Geometry check sheet. Reference: drawing and pictorial views, mm from the part's lowest x, y, z. A direction names the side the tool comes from. Coordinates: 2 decimals unless noted, no trailing zeros. Loops run counter-clockwise (first coordinate to the right, second up) from the corner with the lowest first, then second, coordinate; pieces in that order, holes last.
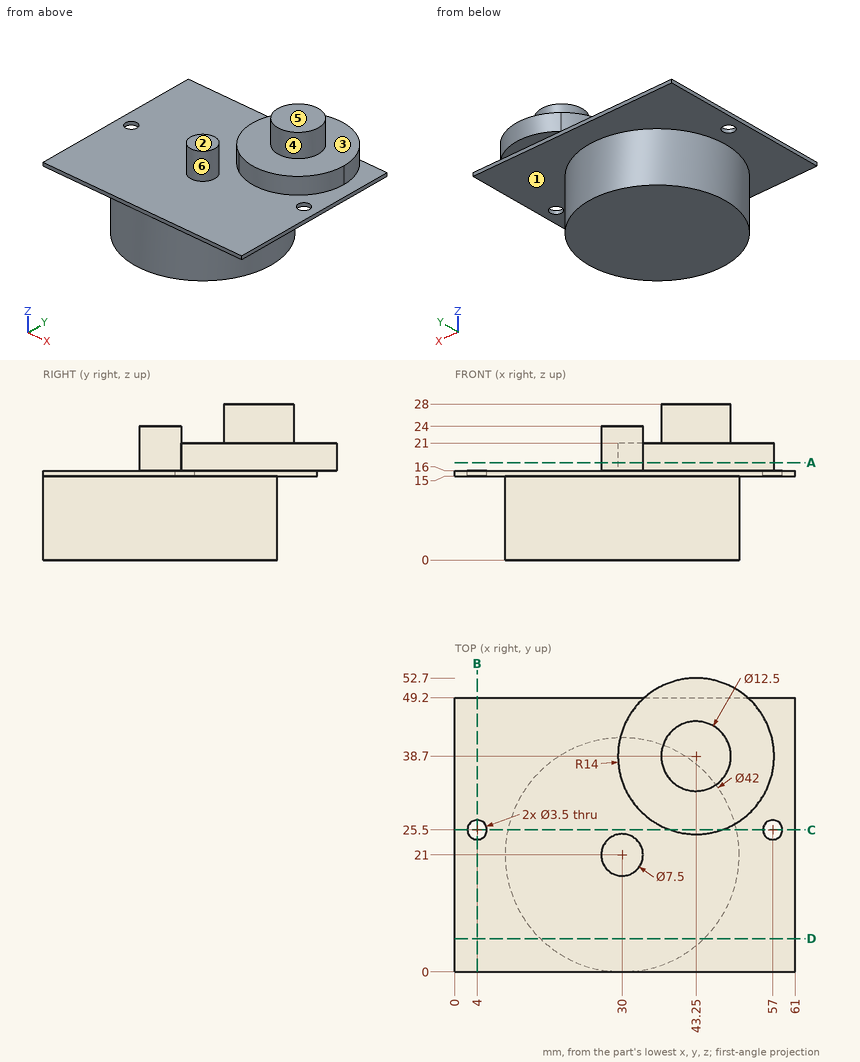
1) Access from +Z, -Z, +X, -X, +Y, -Y to the whole of each face (thin tool, end or side, straight path). Record for the marked faces 1, 2 and 3.
Data:
face 1: -Z
face 2: +Z, +X, -X, +Y, -Y
face 3: +Z
2) Section check A-A on z = 17.5. Record the cut outline in (x, y).
Data:
outline: circle Ø7.5 at (30, 21); circle Ø28 at (43.25, 38.7)
3) Depth check by flat-ended pin: pin 1 (5.5 mm diameter, centred on x = 4, y = 25.5, fed in from -Z); pin 2 (3 mm diameter, centred on x = 13.5, z = 5.5, fed in from +Y); pin 3 (4 mm diameter, centred on x = 57, y = 25.5, fed in from +Z); pin 4 (1.5 mm diameter, centred on y = 12, z = 18, fed in from +X). Enter the tip coordinate at first touch or a pass-through.
Data:
pin 1: stops at z = 15
pin 2: stops at y = 35.7
pin 3: stops at z = 16
pin 4: passes through
4) Section check D-D on y = 6. Record the cut outline in (x, z).
Data:
outline: (0, 15) - (15.3, 15) - (15.3, 0) - (44.7, 0) - (44.7, 15) - (61, 15) - (61, 16) - (0, 16) - close
5) Material ranges on probe 1 along X at (y, z) = (25.5, 15.45); probe 2 along Y at (x, z) = (4, 15.8); probe 3 along X at (y, z) = (21.5, 13), recorded low to high.
Data:
probe 1: x = 0 to 2.25, 5.75 to 55.25, 58.75 to 61
probe 2: y = 0 to 23.75, 27.25 to 49.2
probe 3: x = 9.01 to 50.99
6) Mould release check, pull along Y, two halves, no side actions. Record for the marked faces 4, 5 and 6: +Y half, -Y half, draft (parallel to the pull), parting line (faces both ways), or undercut.
Data:
face 4: parting line
face 5: draft
face 6: undercut
7) Section check C-C on y = 25.5. Record the cut outline in (x, z), and give its area (3 significant figures).
Data:
outline: (0, 15) - (2.25, 15) - (2.25, 16) - (0, 16) - close; (5.75, 15) - (9.49, 15) - (9.49, 0) - (50.51, 0) - (50.51, 15) - (55.25, 15) - (55.25, 16) - (47.91, 16) - (47.91, 21) - (38.59, 21) - (38.59, 16) - (5.75, 16) - close; (58.75, 15) - (61, 15) - (61, 16) - (58.75, 16) - close
area: 716 mm2
8) Section check B-B on x = 4. Record the cut outline in (y, z).
Data:
outline: (0, 15) - (23.75, 15) - (23.75, 16) - (0, 16) - close; (27.25, 15) - (49.2, 15) - (49.2, 16) - (27.25, 16) - close
